from build123d import *

# Parameters (mm, degrees)
SKETCH1_W           = 100
SKETCH1_H           = 100
BOSS_EXTRUDE1_DEPTH = 24
SKETCH2_R           = 6
SKETCH2_R_2         = 7.75
SKETCH2_W           = 25
SKETCH2_H           = 3.6
SKETCH2_W_2         = 13.5
SKETCH2_H_2         = 5.5
CUT_EXTRUDE1_DEPTH  = 22
FILLET1_R           = 7


with BuildPart() as part:
    # Sketch1 → Boss-Extrude1 (new body)
    with BuildSketch(Plane(origin=(0, 0, 0), x_dir=(1, 0, 0), z_dir=(0, 1, 0))):
        Rectangle(SKETCH1_W, SKETCH1_H)
    extrude(amount=BOSS_EXTRUDE1_DEPTH)

    # Sketch2 → Cut-Extrude1 (cut)
    with BuildSketch(Plane(origin=(0, 24, 0), x_dir=(1, 0, 0), z_dir=(0, 1, 0))):
        with Locations(Location((-41, 41, 0), (0, 0, 270))):
            Circle(SKETCH2_R)
        with Locations(Location((-25, 41, 0), (0, 0, 270))):
            Circle(SKETCH2_R)
        with Locations(Location((-9, 41, 0), (0, 0, 270))):
            Circle(SKETCH2_R)
        with Locations(Location((7, 41, 0), (0, 0, 270))):
            Circle(SKETCH2_R)
        with Locations(Location((23, 41, 0), (0, 0, 270))):
            Circle(SKETCH2_R)
        with Locations(Location((39, 41, 0), (0, 0, 270))):
            Circle(SKETCH2_R)
        with Locations(Location((-40, 23, 0), (0, 0, 270))):
            Circle(SKETCH2_R_2)
        with Locations(Location((-20, 23, 0), (0, 0, 270))):
            Circle(SKETCH2_R_2)
        with Locations(Location((0, 23, 0), (0, 0, 270))):
            Circle(SKETCH2_R_2)
        with Locations(Location((20, 23, 0), (0, 0, 270))):
            Circle(SKETCH2_R_2)
        with Locations(Location((40, 23, 0), (0, 0, 270))):
            Circle(SKETCH2_R_2)
        with Locations(Location((-20, 3, 0), (0, 0, 270))):
            Circle(SKETCH2_R_2)
        with Locations(Location((0, 3, 0), (0, 0, 270))):
            Circle(SKETCH2_R_2)
        with Locations(Location((20, 3, 0), (0, 0, 270))):
            Circle(SKETCH2_R_2)
        with Locations(Location((40, 3, 0), (0, 0, 270))):
            Circle(SKETCH2_R_2)
        with Locations(Location((-20, -17, 0), (0, 0, 270))):
            Circle(SKETCH2_R_2)
        with Locations(Location((0, -17, 0), (0, 0, 270))):
            Circle(SKETCH2_R_2)
        with Locations(Location((20, -17, 0), (0, 0, 270))):
            Circle(SKETCH2_R_2)
        with Locations(Location((40, -17, 0), (0, 0, 270))):
            Circle(SKETCH2_R_2)
        with Locations(Location((-40, 3, 0), (0, 0, 270))):
            Circle(SKETCH2_R_2)
        with Locations(Location((-40, -17, 0), (0, 0, 270))):
            Circle(SKETCH2_R_2)
        with Locations((-4.5, -30.8)):
            Rectangle(SKETCH2_W, SKETCH2_H)
        with Locations((-34.5, -30.8)):
            Rectangle(SKETCH2_W, SKETCH2_H)
        with Locations((-4.5, -36.8)):
            Rectangle(SKETCH2_W, SKETCH2_H)
        with Locations((-4.5, -42.8)):
            Rectangle(SKETCH2_W, SKETCH2_H)
        with Locations((-34.5, -36.8)):
            Rectangle(SKETCH2_W, SKETCH2_H)
        with Locations((-34.5, -42.8)):
            Rectangle(SKETCH2_W, SKETCH2_H)
        with Locations((20.25, -31.75)):
            Rectangle(SKETCH2_W_2, SKETCH2_H_2)
        with Locations((40.25, -31.75)):
            Rectangle(SKETCH2_W_2, SKETCH2_H_2)
        with Locations((20.25, -41.75)):
            Rectangle(SKETCH2_W_2, SKETCH2_H_2)
        with Locations((40.25, -41.75)):
            Rectangle(SKETCH2_W_2, SKETCH2_H_2)
    extrude(amount=-CUT_EXTRUDE1_DEPTH, mode=Mode.SUBTRACT)

    # Fillet1
    fillet1_edges = [part.edges().sort_by_distance(p)[0] for p in [
        (50, 12, 50),
        (-50, 12, 50),
        (-50, 12, -50),
        (50, 12, -50),
    ]]
    fillet(fillet1_edges, radius=FILLET1_R)


solid = part.part
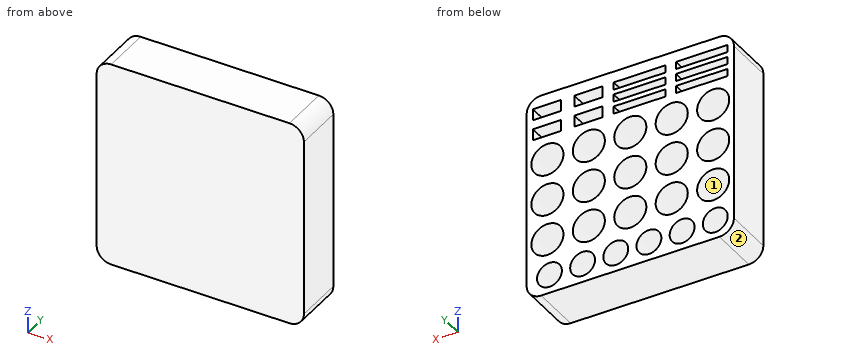
Verification items for the finished model (mm, model axes). Face numbers are marked on the shaded views. A direction names the side the tool comes from. Coordinates: 2 decimals unless noted, no trailing zeros. Write each loop counter-clockwise with the first axis right and the second up, starting at its lowest first coordinate (ties: lowest second). Pieces come first, ordered by that corner, then holes. Notation, with made-up numbers: (-11.75, 14.5) - (25.25, 14.5) arc R21 cw to (25.25, 49.5) - close; hole circle Ø2 at (88, 53). An arc over 180 degrees is marked (long way). Answer as a JSON object with one key per item and string values.
(1) Tool access check on the marked faces 1 and 2. Record the directions out of +Z, -Z, +X, -X, +Y, -Y that give a thin tool (end or side, any length) a straight path to the whole face; none if there is none.
Report:
{"face 1": "+Y", "face 2": "-Z, -X, +Y, -Y"}
(2) Cross-section at C-C on x = -9. Record the cut outline in (y, z).
Report:
{"outline": "(0, -50) - (24, -50) - (24, -47) - (2, -47) - (2, -35) - (24, -35) - (24, 29) - (2, 29) - (2, 32.6) - (24, 32.6) - (24, 35) - (2, 35) - (2, 38.6) - (24, 38.6) - (24, 41) - (2, 41) - (2, 44.6) - (24, 44.6) - (24, 50) - (0, 50) - close"}
(3) Gauge pin test, flat ends, axial feed: pin 1 Ø1.8 at (x, z) = (-38.5, 42.5) entering from +Y; pin 2 Ø8 at (x, z) = (-43, 14.5) entering from +Y. Record the tip position at first contact, or that the pin passes through.
Report:
{"pin 1": "y = 2", "pin 2": "y = 24"}
(4) Cross-section at B-B on y = 22.25. Give the number of separate pieces and of enclosed holes in the cut face, plus the area to 3 significant figures.
Report:
{"separate pieces": "1", "enclosed holes": "31", "area": "5,610 mm^2"}
(5) Cross-section at D-D on z = -23. Record the cut outline in (x, y), plus the area to 3 significant figures.
Report:
{"outline": "(-50, 0) - (50, 0) - (50, 24) - (47.75, 24) - (47.75, 2) - (32.25, 2) - (32.25, 24) - (27.75, 24) - (27.75, 2) - (12.25, 2) - (12.25, 24) - (7.75, 24) - (7.75, 2) - (-7.75, 2) - (-7.75, 24) - (-12.25, 24) - (-12.25, 2) - (-27.75, 2) - (-27.75, 24) - (-32.25, 24) - (-32.25, 2) - (-47.75, 2) - (-47.75, 24) - (-50, 24) - close", "area": "695 mm^2"}
(6) Thickness scan on line 1 along X through (y, z) = (12.75, 32.5); line 2 along X through (y, z) = (13.25, 36); line 3 along X through (y, z) = (15.5, 17). Record the ranges inside material, lowest first.
Report:
{"line 1": "-50 to -47, -22 to -17, 8 to 13.5, 27 to 33.5, 47 to 50", "line 2": "-50 to -47, -22 to -17, 8 to 50", "line 3": "-50 to -47.75, -32.25 to -27.75, -12.25 to -7.75, 7.75 to 12.25, 27.75 to 32.25, 47.75 to 50"}
(7) Cross-section at A-A on z = -41. Record the cut outline in (x, y).
Report:
{"outline": "(-50, 0) - (50, 0) - (50, 24) - (45, 24) - (45, 2) - (33, 2) - (33, 24) - (29, 24) - (29, 2) - (17, 2) - (17, 24) - (13, 24) - (13, 2) - (1, 2) - (1, 24) - (-3, 24) - (-3, 2) - (-15, 2) - (-15, 24) - (-19, 24) - (-19, 2) - (-31, 2) - (-31, 24) - (-35, 24) - (-35, 2) - (-47, 2) - (-47, 24) - (-50, 24) - close"}
